```python
from build123d import *

# Parameters (mm, degrees)
SKETCH_1_R      = 19.858230866
SKETCH_1_R_2    = 11.858230866
EXTRUDE_1_DEPTH = 2
EXTRUDE_3_DEPTH = 0.01


with BuildPart() as part:
    # Эскиз1 → Бобышка-Вытянуть1 (new body)
    with BuildSketch(Plane(origin=(0, 26.1, 0), x_dir=(1, 0, 0), z_dir=(0, 1, 0))):
        with Locations(Location((0, 0, 0), (0, 0, 270))):
            Circle(SKETCH_1_R)
        with Locations(Location((0, 0, 0), (0, 0, 270))):
            Circle(SKETCH_1_R_2, mode=Mode.SUBTRACT)
    extrude(amount=EXTRUDE_1_DEPTH)

    # Эскиз3 → Бобышка-Вытянуть3 (add)
    with BuildSketch(Plane(origin=(0, 28.1, 0), x_dir=(1, 0, 0), z_dir=(0, 1, 0))):
        with BuildLine():
            Line((17.85122992, -0.5), (13.849208019, -0.5))
            ThreePointArc((13.849208019, -0.5), (13.858230866, 0), (13.849208019, 0.5))
            Line((13.849208019, 0.5), (17.85122992, 0.5))
            ThreePointArc((17.85122992, 0.5), (17.858230866, 0), (17.85122992, -0.5))
        make_face()
        with BuildLine():
            Line((17.795123199, -1.5), (13.776812503, -1.5))
            ThreePointArc((13.776812503, -1.5), (-13.858230866, 0), (13.776812503, 1.5))
            Line((13.776812503, 1.5), (17.795123199, 1.5))
            ThreePointArc((17.795123199, 1.5), (-17.858230866, 0), (17.795123199, -1.5))
        make_face()
    extrude(amount=EXTRUDE_3_DEPTH)


solid = part.part
```
The listing builds one solid part. Answer for the finished solid, in the listing's coordinates (mm). Give positions to 0.01 mm unless a question says otherwise; leave off trailing zeros. Order: outer loops, then holes, each group sorted by start corner. A loop starts at its lowest first (then second) coordinate and runs counter-clockwise, first axis right, second up.
Item 1: Given pin 1 Ø1 at (y, z) = (26.5, 15) entering from +X, flat-ended and moving along its own axis, determine where the tip first touches the part or whether it passes through.
From the geometry:
pin 1: stops at x = 13.57
Item 2: Find the intervals of material crossed by probe 1 along Z at (x, y) = (-0.5, 27.45); probe 2 along X at (y, z) = (27.65, 0); probe 3 along Y at (x, z) = (10.5, 7), in increasing order.
From the geometry:
probe 1: z = -19.85 to -11.85, 11.85 to 19.85
probe 2: x = -19.86 to -11.86, 11.86 to 19.86
probe 3: y = 26.1 to 28.1
Item 3: For a pull along X with two mould halves and no side action, classify faces 1 (the face through (5.965, 27.086, 18.941)), 2 (the face through (16, 28.11, 0)), 3 (the face through (-11.576, 27.086, -2.571)) as pulls with the +X half, pulls with the -X half, needs draft (parallel to the pull), parting line crosses it, or undercut.
From the geometry:
face 1: parting line crosses it
face 2: needs draft
face 3: undercut
Item 4: The part is cut by section C-C, the plane y = 27.35. Give the vertices of the cut face in (x, z), and give its area (3 significant figures).
From the geometry:
outline: circle Ø39.72 at (0, 0); hole circle Ø23.72 at (0, 0)
area: 797 mm2
